Geometry: final body of the model. Coordinates: model frame, mm. A direction names the side the tool comes from. Give positions to 0.01 mm unless a question says otherwise; leave off trailing zeros. Write each loop counter-clockwise with the first axis right and the second up, starting at its lowest first coordinate (ties: lowest second). Pieces come first, ordered by that corner, then holes.
Q1. Line query: line 1 (X direction, y = 0, z = -1.75); line 2 (Y direction, x = -3, z = 82.5); line 3 (Y direction, x = 0, z = 45). Output: solid intervals per line, ascending.
Q2. Mould query, pull axis X, two halves, no side actions, for faces 4 (the flat face through (0, 26.91, -2)), 5 (the cylindrical face through (-9.76, -43.93, 86.48)), 6 (the cylindrical face through (-2.17, -9.76, 88.94)). Classes: +X half, -X half, draft (parallel to the pull), parting line (faces both ways), or undercut.
Q3. Section A-A (z = 64). Return the cut outline in (x, y), plus the area to 3 significant figures.
Q4. Reachability of faces 1 (the flat face through (9, 9, 0)), 2 (the cylindrical face through (0.589, -23.086, 91.885)), 3 (the cylindrical face through (-0.867, -3.905, 32.115)) from +Z, -Z, +X, -X, +Y, -Y: full face, straight path, thin tool, end or side. Return the list, or none.
Q5. Section B-B (z = 52.5). Return the cut outline in (x, y).
Q6. Pin query (flat end, axial travel): pin 1 Ø10.5 at (x, y) = (-2, 3.5) entering from -Z; pin 2 Ø10 at (x, z) = (-24, 48.5) entering from -Y; pin 3 Ø1.3 at (x, z) = (0.5, -1.5) entering from +Y. Return the tip coordinate at first contact, or that it passes through.
from build123d import *

# Parameters (mm, degrees)
F3_DEPTH  = 4.9
F4_R      = 20
F4_R_2    = 4
F5_DEPTH  = 4.9
F6_DEPTH  = 8
F7_R      = 5
F9_D      = 5.43
F9_DEPTH  = 1.1
F9_TIP    = 1.6313365807
F10_D     = 5.43
F10_DEPTH = 2.2
F10_TIP   = 1.6313365807
F11_R     = 10.5
F12_DEPTH = 5
F14_DEPTH = 5


with BuildPart() as f2:
    # F0 (on Front) → F2 (revolve)
    with BuildSketch(Plane.XZ):
        with BuildLine():
            Line((4, 0), (25, 0))
            ThreePointArc((25, 0), (25.0633115181, 44.8380443487), (45, 85))
            Line((45, 85), (10, 85))
            ThreePointArc((10, 85), (5.5209994492, 72.8549601322), (4, 60))
            Line((4, 60), (4, 0))
        make_face()
    revolve(axis=Axis((0, 0, 25.1682717353), (0, 0, 1)))

    # F3 (add): a face of the model
    f3_faces = [f2.faces().sort_by_distance(p)[0] for p in [
        (-4.7071067812, 0, 0),
    ]]
    extrude(f3_faces, amount=F3_DEPTH)

    # F4 (on face) → F5 (cut)
    with BuildSketch(Plane(origin=(0, 0, -4.9), x_dir=(1, 0, 0), z_dir=(0, 0, -1))):
        Circle(F4_R)
        Circle(F4_R_2, mode=Mode.SUBTRACT)
    extrude(amount=-F5_DEPTH, mode=Mode.SUBTRACT)

    # F6 (add): a face of the model
    f6_faces = [f2.faces().sort_by_distance(p)[0] for p in [
        (-43.7272077939, 0, 85),
    ]]
    extrude(f6_faces, amount=F6_DEPTH)

    # F7
    f7_edges = [f2.edges().sort_by_distance(p)[0] for p in [
        (-45, 0, 93),
    ]]
    fillet(f7_edges, radius=F7_R)

    # F9
    with Locations(Plane.XY.offset(93)):
        with Locations((14.426644952, 0.1037907432), (-14.573297048, 0)):
            Hole(F9_D / 2, depth=F9_DEPTH)
            with Locations((0, 0, -(F9_DEPTH + F9_TIP / 2))):  # 118° drill point
                Cone(0, F9_D / 2, F9_TIP, mode=Mode.SUBTRACT)

    # F10
    with Locations(Plane.XY.offset(93)):
        with Locations((0, -20.4359735063)):
            Hole(F10_D / 2, depth=F10_DEPTH)
            with Locations((0, 0, -(F10_DEPTH + F10_TIP / 2))):  # 118° drill point
                Cone(0, F10_D / 2, F10_TIP, mode=Mode.SUBTRACT)

    # F11 (on Top) → F12 (cut)
    with BuildSketch(Plane.XY):
        Circle(F11_R)
    extrude(amount=F12_DEPTH, mode=Mode.SUBTRACT)

    # F13 (on face) → F14 (join)
    with BuildSketch(Plane(origin=(0, 0, -4.9), x_dir=(1, 0, 0), z_dir=(0, 0, -1))):
        with BuildLine():
            ThreePointArc((2.125, -24.9095237811), (0, -25), (-2.125, -24.9095237811))
            Line((-2.125, -24.9095237811), (-2.125, -26.9095237811))
            Line((-2.125, -26.9095237811), (2.125, -26.9095237811))
            Line((2.125, -26.9095237811), (2.125, -24.9095237811))
        make_face()
    extrude(amount=-F14_DEPTH)


solid = f2.part
Computed:
1. line 1: x = -25 to -20, 20 to 25
1. line 2: y = -42.9 to -8.28, 8.28 to 42.9
1. line 3: y = -25.1 to -4, 4 to 25.1
2. face 4: draft
2. face 5: parting line
2. face 6: undercut
3. outline: circle Ø63.44 at (0, 0); hole circle Ø8.29 at (0, 0)
3. area: 3,110 mm2
4. face 1: -Z
4. face 2: +Z
4. face 3: +Z, -Z
5. outline: circle Ø54.39 at (0, 0); hole circle Ø8 at (0, 0)
6. pin 1: stops at z = 5
6. pin 2: stops at y = -18.14
6. pin 3: stops at y = 26.91
